Can you work these out from the model? Positions are in its coordinate system, mm. Face numbers are marked on the shaded views. A direction names the side the tool comes from. Coordinates: 2 decimals unless noted, no trailing zeros. Order: outer loops, then holes, each group sorted by start corner. A loop starts at its lowest first (then second) coordinate and runs counter-clockwise, first axis right, second up. Notation, with made-up numbers: (42, 53) - (65, 53) arc R19 ccw to (65, 67) - close; hole circle Ø6 at (52.5, 6). An arc over 180 degrees is marked (long way). Return JSON: item names as keys, results as strings. Group by question number.
1) If I drill on line 1 along Z through (x, y) = (-10, 1.7); line 2 along X through (y, z) = (1.6, -12.5); line 3 along Z through (x, y) = (-10.5, 1.7), over which ranges is the centre line in solid material (lowest first)?
2) Imagine slicing it at B-B (x = -10). Write out the boundary of the cut face in (y, z).
3) Imagine slicing it at A-A (z = -12.5). Write out the boundary of the cut face in (x, y).
4) Which directions (+Z, -Z, +X, -X, +Y, -Y) give clear straight access to the entire face, cutting with the end or side of a thin tool? Please do the marked faces 3 and 4.
5) For pin 1 Ø6 at (x, z) = (-9, -15.5) entering from -Y; pin 2 Ø2.5 at (x, z) = (-9.5, -11.5) entering from +Y, each with a flat end and sliding along its axis, tell me the tip position at first contact or that it passes through.
6) If we mould it in two halves opening along Z, with no side actions, what happens to the marked faces 1 and 2? For each: pulls with the +Z half, pulls with the -Z half, needs draft (parallel to the pull), parting line crosses it, or undercut.
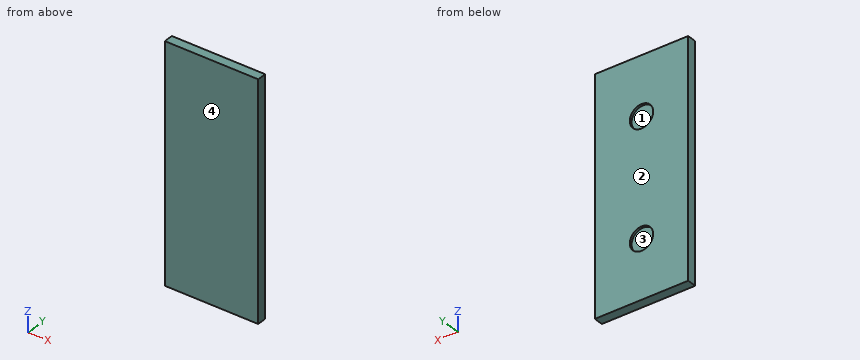
Autodesk Inventor part; units mm, degrees
ref_plane "YZ Plane" through (0, 0, 0) normal (1, 0, 0) x (0, 1, 0)
ref_plane "XZ Plane" through (0, 0, 0) normal (0, 1, 0) x (-1, 0, 0)
ref_plane "XY Plane" through (0, 0, 0) normal (0, 0, 1) x (1, 0, 0)
sketch "Sketch1" plane through (0, 0, 0) normal (0, 1, 0) x (-1, 0, 0)
  line L0 (0, 0) -> (20, 0)
  line L1 (20, 0) -> (20, -50)
  line L2 (20, -50) -> (0, -50)
  line L3 (0, -50) -> (0, 0)
  dimension "d0" = 20
  dimension "d1" = 50
extrude "Extrusion1" add sketch "Sketch1" along normal blind 2
sketch "Sketch2" plane through (0, 2, 0) normal (0, 1, 0) x (1, 0, 0)
  line L0 (-20, 0) -> (0, 0)
  line L1 (-10, 0) -> (-10, 50) construction
  line L2 (0, 50) -> (-20, 50)
  line L3 (-10, 0) -> (-10, 25) construction
  line L4 (-10, 25) -> (-10, 50) construction
  circle A0 centre (-10, 12.5) radius 2.5
  circle A1 centre (-10, 37.5) radius 2.5
  dimension "d4" = 5
  dimension "d5" = 5
extrude "Extrusion2" cut sketch "Sketch2" against normal blind 0.5
properties part number "PortaHerramienta2"
Calculated:
{
 "1": {"line 1": "-50 to -40, -35 to -15, -10 to 0", "line 2": "-20 to -12.5, -7.5 to 0", "line 3": "-50 to -39.95, -35.05 to -14.95, -10.05 to 0"},
 "2": {"outline": "(0, -50) - (2, -50) - (2, -40) - (1.5, -40) - (1.5, -35) - (2, -35) - (2, -15) - (1.5, -15) - (1.5, -10) - (2, -10) - (2, 0) - (0, 0) - close"},
 "3": {"outline": "(-20, 0) - (0, 0) - (0, 2) - (-7.5, 2) - (-7.5, 1.5) - (-12.5, 1.5) - (-12.5, 2) - (-20, 2) - close"},
 "4": {"face 3": "+Y", "face 4": "+Z, -Z, +X, -X, -Y"},
 "5": {"pin 1": "y = 0", "pin 2": "y = 1.5"},
 "6": {"face 1": "undercut", "face 2": "needs draft"}
}
